Geometry check sheet. Reference: the model listing, model coordinates, mm. Face numbers are marked on the shaded views. Coordinates: 2 decimals unless noted, no trailing zeros. Write each loop counter-clockwise with the first axis right and the second up, starting at its lowest first coordinate (ties: lowest second). Pieces come first, ordered by that corner, then holes. Notation, with made-up numbers: M 28.5,25 L 74.5,25 A20 ccw 74.5,60 Z; hole C 70.25,76.25 d1. An arc over 180 degrees is marked long. Write item = value, one per line. Start each with the question number.
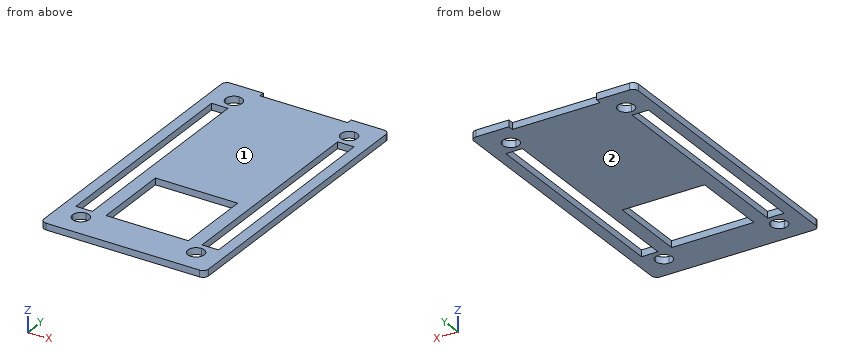
```python
from build123d import *

# Parameters (mm, degrees)
F0_W     = 4
F0_H     = 1
F0_W_2   = 2
F0_H_2   = 39
F0_W_3   = 2.5
F0_H_3   = 0.8
F0_W_4   = 7.5
F0_W_5   = 0.5
F1_DEPTH = 1.2


with BuildPart() as f1:
    # F0 (on Top) → F1 (new body)
    with BuildSketch(Plane.XY):
        with BuildLine():
            Line((-13, 24.5), (-12, 24.5))
            Line((-12, 24.5), (-10.5, 24.5))
            Line((-10.5, 24.5), (-8, 24.5))
            Line((-8, 24.5), (-8, 25.5))
            Line((-8, 25.5), (-8, 26.5))
            Line((-8, 26.5), (-14, 26.5))
            ThreePointArc((-14, 26.5), (-14.7071067812, 26.2071067812), (-15, 25.5))
            Line((-15, 25.5), (-15, 19.5))
            Line((-15, 19.5), (-13, 19.5))
            Line((-13, 19.5), (-13, 22))
            Line((-13, 22), (-13, 23.5))
            Line((-13, 23.5), (-13, 24.5))
        make_face()
        with BuildLine():
            Line((-10.5, 24.5), (-12, 24.5))
            ThreePointArc((-12, 24.5), (-12.7071067812, 24.2071067812), (-13, 23.5))
            Line((-13, 23.5), (-13, 22))
            Line((-13, 22), (-12, 22))
            ThreePointArc((-12, 22), (-11.5606601718, 23.0606601718), (-10.5, 23.5))
            Line((-10.5, 23.5), (-10.5, 24.5))
        make_face()
        with BuildLine():
            ThreePointArc((-13, 23.5), (-12.7071067812, 24.2071067812), (-12, 24.5))
            Line((-12, 24.5), (-13, 24.5))
            Line((-13, 24.5), (-13, 23.5))
        make_face()
        with BuildLine():
            Line((-8, 24.5), (-10.5, 24.5))
            Line((-10.5, 24.5), (-10.5, 23.5))
            ThreePointArc((-10.5, 23.5), (-9.4393398282, 23.0606601718), (-9, 22))
            ThreePointArc((-9, 22), (-9.4393398282, 20.9393398282), (-10.5, 20.5))
            Line((-10.5, 20.5), (-10.5, 19.5))
            Line((-10.5, 19.5), (-10, 19.5))
            Line((-10, 19.5), (10, 19.5))
            Line((10, 19.5), (10.5, 19.5))
            Line((10.5, 19.5), (10.5, 20.5))
            ThreePointArc((10.5, 20.5), (9, 22), (10.5, 23.5))
            Line((10.5, 23.5), (10.5, 24.5))
            Line((10.5, 24.5), (8, 24.5))
            Line((8, 24.5), (4, 24.5))
            Line((4, 24.5), (4, 20))
            Line((4, 20), (-4, 20))
            Line((-4, 20), (-4, 24.5))
            Line((-4, 24.5), (-8, 24.5))
        make_face()
        with Locations((-6, 25)):
            Rectangle(F0_W, F0_H)
        with BuildLine():
            Line((-12, 22), (-13, 22))
            Line((-13, 22), (-13, 19.5))
            Line((-13, 19.5), (-10.5, 19.5))
            Line((-10.5, 19.5), (-10.5, 20.5))
            ThreePointArc((-10.5, 20.5), (-11.5606601718, 20.9393398282), (-12, 22))
        make_face()
        with Locations((-2, 25)):
            Rectangle(F0_W, F0_H)
        Polygon((0, 24.5), (-4, 24.5), (-4, 20), (4, 20), (4, 24.5), align=None)
        with Locations((-14, 0)):
            Rectangle(F0_W_2, F0_H_2)
        with Locations((2, 25)):
            Rectangle(F0_W, F0_H)
        with Locations((-11.75, -19.9)):
            Rectangle(F0_W_3, F0_H_3)
        with Locations((-14, -19.9)):
            Rectangle(F0_W_2, F0_H_3)
        with Locations((6, 25)):
            Rectangle(F0_W, F0_H)
        with BuildLine():
            Line((-10.5, -20.3), (-13, -20.3))
            Line((-13, -20.3), (-13, -22))
            Line((-13, -22), (-12, -22))
            ThreePointArc((-12, -22), (-11.5606601718, -20.9393398282), (-10.5, -20.5))
            Line((-10.5, -20.5), (-10.5, -20.3))
        make_face()
        with BuildLine():
            Line((-13, -22), (-13, -20.3))
            Line((-13, -20.3), (-15, -20.3))
            Line((-15, -20.3), (-15, -25.5))
            ThreePointArc((-15, -25.5), (-14.7071067812, -26.2071067812), (-14, -26.5))
            Line((-14, -26.5), (14, -26.5))
            ThreePointArc((14, -26.5), (14.7071067812, -26.2071067812), (15, -25.5))
            Line((15, -25.5), (15, -20.3))
            Line((15, -20.3), (13, -20.3))
            Line((13, -20.3), (13, -22))
            Line((13, -22), (13, -23.5))
            ThreePointArc((13, -23.5), (12.7071067812, -24.2071067812), (12, -24.5))
            Line((12, -24.5), (10.5, -24.5))
            Line((10.5, -24.5), (-10.5, -24.5))
            Line((-10.5, -24.5), (-12, -24.5))
            ThreePointArc((-12, -24.5), (-12.7071067812, -24.2071067812), (-13, -23.5))
            Line((-13, -23.5), (-13, -22))
        make_face()
        Polygon((-10, -19.5), (-10.5, -19.5), (-10.5, -20.3), (-7.5, -20.3), (-7.5, -19.5), align=None)
        Polygon((10, 19.5), (-10, 19.5), (-10, -19.5), (-7.5, -19.5), (-7.5, -5.3), (7.5, -5.3), (7.5, -19.5), (10, -19.5), (10, 19.1765315831), align=None)
        with BuildLine():
            Line((8, 25.5), (8, 24.5))
            Line((8, 24.5), (10.5, 24.5))
            Line((10.5, 24.5), (12, 24.5))
            ThreePointArc((12, 24.5), (12.7071067812, 24.2071067812), (13, 23.5))
            Line((13, 23.5), (13, 22))
            Line((13, 22), (13, 19.5))
            Line((13, 19.5), (15, 19.5))
            Line((15, 19.5), (15, 25.5))
            ThreePointArc((15, 25.5), (14.7071067812, 26.2071067812), (14, 26.5))
            Line((14, 26.5), (8, 26.5))
            Line((8, 26.5), (8, 25.5))
        make_face()
        with BuildLine():
            Line((-12, -22), (-13, -22))
            Line((-13, -22), (-13, -23.5))
            ThreePointArc((-13, -23.5), (-12.7071067812, -24.2071067812), (-12, -24.5))
            Line((-12, -24.5), (-10.5, -24.5))
            Line((-10.5, -24.5), (-10.5, -23.5))
            ThreePointArc((-10.5, -23.5), (-11.5606601718, -23.0606601718), (-12, -22))
        make_face()
        with BuildLine():
            Line((-7.5, -20.3), (-10.5, -20.3))
            Line((-10.5, -20.3), (-10.5, -20.5))
            ThreePointArc((-10.5, -20.5), (-9.4393398282, -20.9393398282), (-9, -22))
            ThreePointArc((-9, -22), (-9.4393398282, -23.0606601718), (-10.5, -23.5))
            Line((-10.5, -23.5), (-10.5, -24.5))
            Line((-10.5, -24.5), (10.5, -24.5))
            Line((10.5, -24.5), (10.5, -23.5))
            ThreePointArc((10.5, -23.5), (9, -22), (10.5, -20.5))
            Line((10.5, -20.5), (10.5, -20.3))
            Line((10.5, -20.3), (10, -20.3))
            Line((10, -20.3), (7.5, -20.3))
            Line((7.5, -20.3), (0, -20.3))
            Line((0, -20.3), (-7.5, -20.3))
        make_face()
        with BuildLine():
            Line((12, 24.5), (10.5, 24.5))
            Line((10.5, 24.5), (10.5, 23.5))
            ThreePointArc((10.5, 23.5), (11.5606601718, 23.0606601718), (12, 22))
            Line((12, 22), (13, 22))
            Line((13, 22), (13, 23.5))
            ThreePointArc((13, 23.5), (12.7071067812, 24.2071067812), (12, 24.5))
        make_face()
        with Locations((-3.75, -19.9)):
            Rectangle(F0_W_4, F0_H_3)
        with BuildLine():
            Line((10.5, 20.5), (10.5, 19.5))
            Line((10.5, 19.5), (13, 19.5))
            Line((13, 19.5), (13, 22))
            Line((13, 22), (12, 22))
            ThreePointArc((12, 22), (11.5606601718, 20.9393398282), (10.5, 20.5))
        make_face()
        with Locations((3.75, -19.9)):
            Rectangle(F0_W_4, F0_H_3)
        with Locations((8.75, -19.9)):
            Rectangle(F0_W_3, F0_H_3)
        with Locations((10.25, -19.9)):
            Rectangle(F0_W_5, F0_H_3)
        with Locations((14, 0)):
            Rectangle(F0_W_2, F0_H_2)
        with Locations((11.75, -19.9)):
            Rectangle(F0_W_3, F0_H_3)
        with Locations((14, -19.9)):
            Rectangle(F0_W_2, F0_H_3)
        with BuildLine():
            Line((10.5, -23.5), (10.5, -24.5))
            Line((10.5, -24.5), (12, -24.5))
            ThreePointArc((12, -24.5), (12.7071067812, -24.2071067812), (13, -23.5))
            Line((13, -23.5), (13, -22))
            Line((13, -22), (12, -22))
            ThreePointArc((12, -22), (11.5606601718, -23.0606601718), (10.5, -23.5))
        make_face()
        with BuildLine():
            Line((13, -20.3), (10.5, -20.3))
            Line((10.5, -20.3), (10.5, -20.5))
            ThreePointArc((10.5, -20.5), (11.5606601718, -20.9393398282), (12, -22))
            Line((12, -22), (13, -22))
            Line((13, -22), (13, -20.3))
        make_face()
    extrude(amount=F1_DEPTH)


solid = f1.part
```
Q1. Draft check along Z on the marked faces 1 and 2. Enter one of: pulls with the +Z half, pulls with the -Z half, needs draft (parallel to the pull), parting line crosses it, or undercut.
Q2. Cross-section at C-C on y = -8. Enter the section's corners in (x, z), and give its area (3 significant figures).
Q3. Cross-section at B-B on x = 4.25. Enter the section's corners in (y, z), and give its area (3 significant figures).
Q4. Scan lines: L1, parallel to X at y = 15, z = 1; L2, parallel to X at y = -18, z = 0.1; L3, parallel to Y at x = 5.5, z = 0.7. Record each from-to range of solid material in increasing order.
Q5. Cross-section at A-A on y = 0.5. Enter the section's corners in (x, z), and give its area (3 significant figures).
Q6. Cross-section at D-D on z = 0.7. Enter the section's corners in (x, y), and give its area (3 significant figures).
Q7. Gauge pin test, flat end, axial feed: pin 1 (1.5 mm diameter, centred on x = -1.5, y = 10, fed in from -Z). Record the tip position at first contact, or that the pin passes through.
Values found:
q1.face_1 = pulls with the +Z half
q1.face_2 = pulls with the -Z half
q2.outline = M -15,0 L -13,0 L -13,1.2 L -15,1.2 Z; M -10,0 L -7.5,0 L -7.5,1.2 L -10,1.2 Z; M 7.5,0 L 10,0 L 10,1.2 L 7.5,1.2 Z; M 13,0 L 15,0 L 15,1.2 L 13,1.2 Z
q2.area = 10.8 mm²
q3.outline = M -26.5,0 L -19.5,0 L -19.5,1.2 L -26.5,1.2 Z; M -5.3,0 L 25.5,0 L 25.5,1.2 L -5.3,1.2 Z
q3.area = 45.4 mm²
q4.L1 = -15 to -13, -10 to 10, 13 to 15
q4.L2 = -15 to -13, -10 to -7.5, 7.5 to 10, 13 to 15
q4.L3 = -26.5 to -19.5, -5.3 to 25.5
q5.outline = M -15,0 L -13,0 L -13,1.2 L -15,1.2 Z; M -10,0 L 10,0 L 10,1.2 L -10,1.2 Z; M 13,0 L 15,0 L 15,1.2 L 13,1.2 Z
q5.area = 28.8 mm²
q6.outline = M -15,-25.5 A1 ccw -14,-26.5 L 14,-26.5 A1 ccw 15,-25.5 L 15,25.5 A1 ccw 14,26.5 L 8,26.5 L 8,25.5 L -8,25.5 L -8,26.5 L -14,26.5 A1 ccw -15,25.5 Z; hole M -13,-19.5 L -10,-19.5 L -10,19.5 L -13,19.5 Z; hole C -10.5,-22 d3; hole C -10.5,22 d3; hole M -7.5,-19.5 L 7.5,-19.5 L 7.5,-5.3 L -7.5,-5.3 Z; hole C 10.5,-22 d3; hole C 10.5,22 d3; hole M 10,-19.5 L 13,-19.5 L 13,19.5 L 10,19.5 Z
q6.area = 1,100 mm²
q7.pin_1 = 0
